Design review of the part built by this model. Coordinates are the model's own, in mm. Face numbers are marked on the shaded views. A direction names the side the tool comes from. Coordinates: 2 decimals unless noted, no trailing zeros. Loops run counter-clockwise (first coordinate to the right, second up) from the corner with the lowest first, then second, coordinate; pieces in that order, holes last. Notation, with made-up numbers: (-13.5, -4.5) - (10.5, -4.5) arc R37 cw to (10.5, 32.5) - close; hole circle Ø6 at (-19.75, 30). An arc over 180 degrees is marked (long way). Use one line per item in the form item = value. Start each with the question number.
(1) Add section C-C (x = 20.5). State the section outline as (y, z) points, plus the area to 3 significant figures.
(2) Clearance check with flat-ended pins moving along their axes: pin 1 Ø4 at (y, z) = (1.5, -7.5) entering from +X; pin 2 Ø2 at (y, z) = (4, -10.5) entering from +X; pin 3 Ø2 at (x, z) = (-7, 2) entering from +Y; pin 4 Ø3.5 at (x, z) = (96.87, 1.23) entering from +Y. State where each tip first meets the part, or that it passes through.
(3) For L1, parallel to X at y = 8, z = -1.75; L2, parallel to Z at x = -14.5, y = 1.75; L3, parallel to Z at x = 56, y = 4.25, list the stretches that pass through material, from the lowest coordinate up.
(4) Tool access review of the marked faces 1, 2, 3 and 4: name each direction out of +Z, -Z, +X, -X, +Y, -Y from which nothing blocks a thin tool from reaching the whole face with its end or side.
(5) Add section B-B (x = -4). State the section outline as (y, z) points, plus the area to 3 significant figures.
(6) Add section A-A (x = 64). State the section outline as (y, z) points, plus the area to 3 significant figures.
```python
from build123d import *

# Parameters (mm, degrees)
F0_W         = 50.8
F0_H         = 19.7104
F0_W_2       = 43.18
F0_H_2       = 10
F0_H_3       = 12.7
F1_DEPTH     = 10.16
F2_W         = 50.8
F2_H         = 3.6068
F2_H_2       = 19.7104
F3_DEPTH     = 3.048
F4_W         = 45.72
F4_H         = 9.652
F4_W_2       = 2.54
F4_H_2       = 6.952
F4_W_3       = 12.7
F5_DEPTH     = 8.128
F8_DEPTH     = 25
F10_T1_DEPTH = 25.16
F10_T3_DEPTH = 17.032
F12_D        = 1.6
F12_DEPTH    = 5.842
F12_TIP      = 0.4806884952
F13_W        = 5.715
F13_H        = 3.6068
F14_DEPTH    = 2.54
F15_W        = 5.715
F15_H        = 3.6068
F16_DEPTH    = 2.54
F17_DEPTH    = 25.4
F18_R        = 2.54
F20_D        = 3.81
F21_W        = 6.35
F21_H        = 9.652
F22_W        = 6.35
F22_H        = 6.952
F23_DEPTH    = 8.128
F25_D        = 3.2639
F25_DEPTH    = 8.255
F25_TIP      = 0.9805744872


# Not quite as in the source:
# - a fillet or chamfer that OpenCascade refuses, or shapes differently, is made with other operations: its cross-section is extruded or revolved along the edge and cut away or added


with BuildPart() as f1:
    # F0 (on Front) → F1 (new body)
    with BuildSketch(Plane.XZ):
        Polygon((75.1493134361, 16.2306381539), (19.2693134361, 16.2306381539), (19.2693134361, 6.2332381539), (19.2693134361, -3.7667618461), (19.2693134361, -13.7667618461), (75.1493134361, -13.7667618461), (75.1493134361, -5.1180618461), (75.1493134361, 7.5819381539), align=None)
        with Locations((47.2093134361, 1.2319381539)):
            Rectangle(F0_W, F0_H, mode=Mode.SUBTRACT)
        with Locations((-2.3206865639, 1.2332381539)):
            Rectangle(F0_W_2, F0_H_2)
        with Locations((96.7393134361, 1.2319381539)):
            Rectangle(F0_W_2, F0_H_3)
    extrude(amount=-F1_DEPTH)

    # F2 (on face) → F3 (cut)
    with BuildSketch(Plane(origin=(0, 10.16, 0), x_dir=(-1, 0, 0), z_dir=(0, 1, 0))):
        with Locations((-47.2093134361, -10.4266618461)):
            Rectangle(F2_W, F2_H)
        with Locations((-47.2093134361, 1.2319381539)):
            Rectangle(F2_W, F2_H_2)
        with Locations((-47.2093134361, 12.8905381539)):
            Rectangle(F2_W, F2_H)
    extrude(amount=-F3_DEPTH, mode=Mode.SUBTRACT)

    # F4 (on face) → F5 (cut)
    with BuildSketch(Plane(origin=(0, 10.16, 0), x_dir=(-1, 0, 0), z_dir=(0, 1, 0))):
        with Locations((-95.4693134361, 1.2319381539)):
            Rectangle(F4_W, F4_H)
        with Locations((-71.3393134361, 1.2319381539)):
            Rectangle(F4_W_2, F4_H)
        with Locations((-23.0793134361, 1.2332381539)):
            Rectangle(F4_W_2, F4_H_2)
        with Locations((1.0506865639, 1.2332381539)):
            Rectangle(F4_W, F4_H_2)
        with Locations((30.2606865639, 1.2332381539)):
            Rectangle(F4_W_3, F4_H_2)
    extrude(amount=-F5_DEPTH, mode=Mode.SUBTRACT)

    # F7 (on face) + F6 (on face) → F8 (cut)
    with BuildSketch(Plane.XY.offset(6.2332381539)):
        Polygon((-23.9106865639, 10.16), (-23.9106865639, 2.032), (-12.0996865639, 10.16), align=None)
    with BuildSketch(Plane.XY.offset(7.5819381539)):
        Polygon((118.3293134361, 10.16), (106.5183134361, 10.16), (118.3293134361, 2.032), align=None)
    extrude(amount=-F8_DEPTH, mode=Mode.SUBTRACT)

    # F10: fillet of radius 3 on 8 edges, made by hand

    # F10_s2 → F10_t1 (cut)
    with BuildSketch(Plane.XZ.offset(-17.66)):
        with BuildLine():
            ThreePointArc((72.1493134361, -13.7667618461), (74.2706337797, -12.8880821896), (75.1493134361, -10.7667618461))
            Line((75.1493134361, -10.7667618461), (75.1493134361, -13.7667618461))
            Line((75.1493134361, -13.7667618461), (72.1493134361, -13.7667618461))
        make_face()
        with BuildLine():
            ThreePointArc((19.2693134361, -10.7667618461), (20.1479930925, -12.8880821896), (22.2693134361, -13.7667618461))
            Line((22.2693134361, -13.7667618461), (19.2693134361, -13.7667618461))
            Line((19.2693134361, -13.7667618461), (19.2693134361, -10.7667618461))
        make_face()
        with BuildLine():
            ThreePointArc((22.2693134361, 16.2306381539), (20.1479930925, 15.3519584975), (19.2693134361, 13.2306381539))
            Line((19.2693134361, 13.2306381539), (19.2693134361, 16.2306381539))
            Line((19.2693134361, 16.2306381539), (22.2693134361, 16.2306381539))
        make_face()
        with BuildLine():
            ThreePointArc((72.1493134361, 16.2306381539), (74.2706337797, 15.3519584975), (75.1493134361, 13.2306381539))
            Line((75.1493134361, 13.2306381539), (75.1493134361, 16.2306381539))
            Line((75.1493134361, 16.2306381539), (72.1493134361, 16.2306381539))
        make_face()
    extrude(amount=F10_T1_DEPTH, mode=Mode.SUBTRACT)

    # F10_s4 → F10_t3 (cut)
    with BuildSketch(Plane.XZ.offset(-9.532)):
        with BuildLine():
            ThreePointArc((-23.9106865639, -0.7667618461), (-23.0320069075, -2.8880821896), (-20.9106865639, -3.7667618461))
            Line((-20.9106865639, -3.7667618461), (-23.9106865639, -3.7667618461))
            Line((-23.9106865639, -3.7667618461), (-23.9106865639, -0.7667618461))
        make_face()
        with BuildLine():
            ThreePointArc((-20.9106865639, 6.2332381539), (-23.0320069075, 5.3545584975), (-23.9106865639, 3.2332381539))
            Line((-23.9106865639, 3.2332381539), (-23.9106865639, 6.2332381539))
            Line((-23.9106865639, 6.2332381539), (-20.9106865639, 6.2332381539))
        make_face()
        with BuildLine():
            ThreePointArc((115.3293134361, -5.1180618461), (117.4506337797, -4.2393821896), (118.3293134361, -2.1180618461))
            Line((118.3293134361, -2.1180618461), (118.3293134361, -5.1180618461))
            Line((118.3293134361, -5.1180618461), (115.3293134361, -5.1180618461))
        make_face()
        with BuildLine():
            ThreePointArc((115.3293134361, 7.5819381539), (117.4506337797, 6.7032584975), (118.3293134361, 4.5819381539))
            Line((118.3293134361, 4.5819381539), (118.3293134361, 7.5819381539))
            Line((118.3293134361, 7.5819381539), (115.3293134361, 7.5819381539))
        make_face()
    extrude(amount=F10_T3_DEPTH, mode=Mode.SUBTRACT)

    # F12
    with Locations(Plane(origin=(0, 7.112, 0), x_dir=(-1, 0, 0), z_dir=(0, 1, 0))):
        with Locations((-68.9771134361, 12.5857381539), (-25.4415134361, 12.5870381539), (-25.4415134361, -10.1205618461), (-68.9771134361, -10.1218618461)):
            Hole(F12_D / 2, depth=F12_DEPTH)
            with Locations((0, 0, -(F12_DEPTH + F12_TIP / 2))):  # 118° drill point
                Cone(0, F12_D / 2, F12_TIP, mode=Mode.SUBTRACT)

    # F13 (on face) → F14 (cut)
    with BuildSketch(Plane(origin=(0, 7.112, 0), x_dir=(-1, 0, 0), z_dir=(0, 1, 0))):
        with Locations((-50.0668134361, 12.8905381539)):
            Rectangle(F13_W, F13_H)
        with Locations((-44.3518134361, 12.8905381539)):
            Rectangle(F13_W, F13_H)
    extrude(amount=-F14_DEPTH, mode=Mode.SUBTRACT)

    # F15 (on face) → F16 (cut)
    with BuildSketch(Plane(origin=(0, 7.112, 0), x_dir=(-1, 0, 0), z_dir=(0, 1, 0))):
        with Locations((-50.0668134361, -10.4266618461)):
            Rectangle(F15_W, F15_H)
        with Locations((-44.3518134361, -10.4266618461)):
            Rectangle(F15_W, F15_H)
    extrude(amount=-F16_DEPTH, mode=Mode.SUBTRACT)

    # F9 (on face) → F17 (cut)
    with BuildSketch(Plane(origin=(0, 2.032, 0), x_dir=(-1, 0, 0), z_dir=(0, 1, 0))):
        with BuildLine():
            Line((-112.8048134361, -0.8584618461), (-108.6138134361, -0.8584618461))
            ThreePointArc((-108.6138134361, -0.8584618461), (-106.5183134361, 1.2370381539), (-108.6138134361, 3.3325381539))
            Line((-108.6138134361, 3.3325381539), (-112.8048134361, 3.3325381539))
            ThreePointArc((-112.8048134361, 3.3325381539), (-114.9003134361, 1.2370381539), (-112.8048134361, -0.8584618461))
        make_face()
        with BuildLine():
            Line((18.3861865639, 3.3325381428), (14.1951865639, 3.3325381428))
            ThreePointArc((14.1951865639, 3.3325381428), (12.0996865639, 1.2370381428), (14.1951865639, -0.8584618572))
            Line((14.1951865639, -0.8584618572), (18.3861865639, -0.8584618572))
            ThreePointArc((18.3861865639, -0.8584618572), (20.4816865639, 1.2370381428), (18.3861865639, 3.3325381428))
        make_face()
    extrude(amount=-F17_DEPTH, mode=Mode.SUBTRACT)

    # F18
    f18_edges = [f1.edges().sort_by_distance(p)[0] for p in [
        (75.149313, 5.08, 7.581938),
        (75.149313, 5.08, -5.118062),
        (19.269313, 5.08, 6.233238),
        (19.269313, 5.08, -3.766762),
    ]]
    fillet(f18_edges, radius=F18_R)

    # F20 (through all)
    with Locations(Plane(origin=(0, 2.032, 0), x_dir=(-1, 0, 0), z_dir=(0, 1, 0))):
        with Locations((-101.9463134361, 1.2319381539), (-91.7863134361, 1.2319381539), (-81.6263134361, 1.2319381539), (-86.7063134361, 1.2319381539), (-96.8663134361, 1.2319381539)):
            Hole(F20_D / 2)

    # F21 (on face) + F22 (on face) → F23 (join)
    with BuildSketch(Plane(origin=(0, 2.032, 0), x_dir=(-1, 0, 0), z_dir=(0, 1, 0))):
        with Locations((-75.7843134361, 1.2319381539)):
            Rectangle(F21_W, F21_H)
    with BuildSketch(Plane(origin=(0, 2.032, 0), x_dir=(-1, 0, 0), z_dir=(0, 1, 0))):
        with Locations((-18.6343134361, 1.2332381539)):
            Rectangle(F22_W, F22_H)
    extrude(amount=F23_DEPTH)

    # F25
    with Locations(Plane(origin=(0, 0, -5.1180618461), x_dir=(1, 0, 0), z_dir=(0, 0, -1))):
        with Locations((84.1663134361, -6.223), (99.4063134361, -6.223)):
            Hole(F25_D / 2, depth=F25_DEPTH)
            with Locations((0, 0, -(F25_DEPTH + F25_TIP / 2))):  # 118° drill point
                Cone(0, F25_D / 2, F25_TIP, mode=Mode.SUBTRACT)


solid = f1.part
```
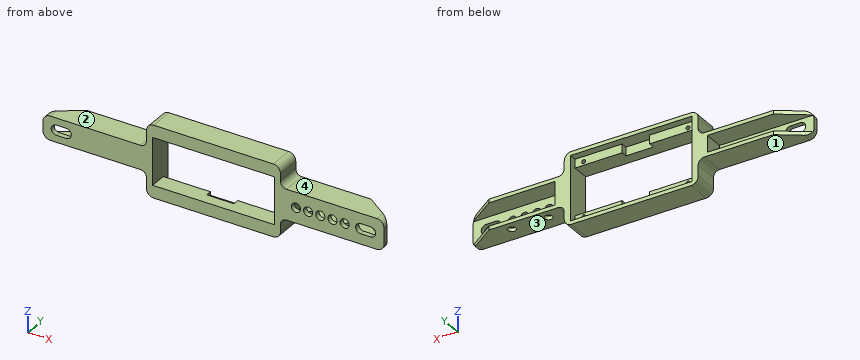
Computed values:
q1.outline = (0, -13.19) - (10.16, -13.19) - (10.16, 15.65) - (0, 15.65) - close
q1.area = 293 mm^2
q2.pin_1 = 76.35
q2.pin_2 = 75.15
q2.pin_3 = 2.03
q2.pin_4 = through
q3.L1 = 15.46 to 21.81, 72.61 to 78.96
q3.L2 = -3.77 to -0.86, 3.33 to 6.23
q3.L3 = -13.77 to -8.62, 11.09 to 16.23
q4.face_1 = -Z, -X, +Y, -Y
q4.face_2 = +Z, -X, +Y, -Y
q4.face_3 = -Z, +X, +Y, -Y
q4.face_4 = +Z, +X, +Y, -Y
q5.outline = (0, -3.77) - (10.16, -3.77) - (10.16, -2.24) - (2.03, -2.24) - (2.03, 4.71) - (10.16, 4.71) - (10.16, 6.23) - (0, 6.23) - close
q5.area = 45.1 mm^2
q6.outline = (0, -13.77) - (10.16, -13.77) - (10.16, -12.23) - (7.11, -12.23) - (7.11, -8.62) - (0, -8.62) - close; (0, 11.09) - (7.11, 11.09) - (7.11, 14.69) - (10.16, 14.69) - (10.16, 16.23) - (0, 16.23) - close
q6.area = 82.5 mm^2
